Can you work these out from the model? Positions are in its coordinate system, mm. Round coordinates to 2 decimals unless told otherwise and drop trailing zeros. Loops run counter-clockwise (first coordinate to the right, second up) from the corner with the lowest first, then second, coordinate; pieces in that order, holes last. Notation, with made-up numbers: (36.5, -24) -> (57.5, -24) arc R21 cw to (57.5, 9) -> close; hole circle Ø4 at (11.25, -26.75). An arc over 180 degrees is marked (long way). Use a Markdown table: item, result.
from build123d import *

# Parameters (mm, degrees)
F1_DEPTH       = 400
F3_SIZE        = 4
F5_DEPTH       = 8.5
F6_D           = 5.5
F6_CBORE_D     = 10
F6_CBORE_DEPTH = 5


with BuildPart() as f1:
    # F0 (on Top) → F1 (new body)
    with BuildSketch(Plane.XY):
        Polygon((4.216131, -6.269906), (-15.783869, -6.269906), (-15.783869, -18.269906), (-0.783869, -18.269906), (-0.783869, -9.769906), (4.216131, -9.769906), align=None)
    extrude(amount=F1_DEPTH)

    # F3
    f3_edges = [f1.edges().sort_by_distance(p)[0] for p in [
        (4.216131, -8.019906, 400),
        (4.216131, -8.019906, 0),
    ]]
    chamfer(f3_edges, length=F3_SIZE)

    # F4 (on face) → F5 (cut)
    with BuildSketch(Plane.XZ.offset(18.269906)):
        Polygon((-0.783869, 392), (-0.783869, 400), (-5.402671, 400), align=None)
        Polygon((-0.783869, 0), (-0.783869, 8), (-5.402671, 0), align=None)
    extrude(amount=-F5_DEPTH, mode=Mode.SUBTRACT)

    # F6 (through all)
    with Locations(Plane(origin=(0, -6.269906, 0), x_dir=(-1, 0, 0), z_dir=(0, 1, 0))):
        with Locations((8.283869, 15.1), (8.283869, 138.4), (8.283869, 261.7), (8.283869, 385)):
            CounterBoreHole(F6_D / 2, F6_CBORE_D / 2, F6_CBORE_DEPTH)


solid = f1.part
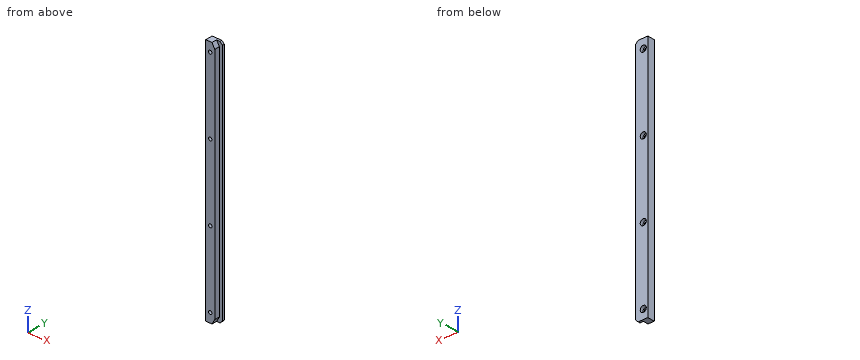
1. I need wall thicknesses on line 1 (Z direction, x = -7.75, y = -12.25); line 2 (X direction, y = -15, z = 138.4); line 3 (Z direction, x = -7.5, y = -11.75). Which ranges of each line are inside material? Lowest first, please.
Answer sheet:
| item | result |
|---|---|
| line 1 | z = 0 to 12.4, 17.8 to 135.7, 141.1 to 259, 264.4 to 382.3, 387.7 to 400 |
| line 2 | x = -15.78 to -11.03, -5.53 to -0.78 |
| line 3 | z = 0 to 12.46, 17.74 to 135.76, 141.04 to 259.06, 264.34 to 382.36, 387.64 to 400 |
2. I want a section at A-A (z = 240.5). Please give me the cut outline in (x, y), plus the area to 4 significant figures.
Answer sheet:
| item | result |
|---|---|
| outline | (-15.78, -18.27) -> (-0.78, -18.27) -> (-0.78, -9.77) -> (4.22, -9.77) -> (4.22, -6.27) -> (-15.78, -6.27) -> close |
| area | 197.5 mm² |
3. Will these pins go through, and if not, where does the flat tip stop? pin 1 Ø5 at (x, z) = (-8.28, 15.1) entering from -Y; pin 2 Ø5 at (x, z) = (-8, 139.5) entering from +Y; pin 3 Ø5 at (x, y) = (-3.5, -10.5) entering from -Z; pin 4 Ø6 at (y, z) = (-16, 300) entering from +X.
Answer sheet:
| item | result |
|---|---|
| pin 1 | passes through |
| pin 2 | stops at y = -11.27 |
| pin 3 | stops at z = 0 |
| pin 4 | stops at x = -0.78 |
